from build123d import *

# Parameters (mm, degrees)
BOSS_EXTRUDE1_DEPTH = 50.8
CUT_EXTRUDE1_REACH  = 61.906
SKETCH2_R           = 3.175
CUT_EXTRUDE2_REACH  = 61.906
SKETCH3_R           = 3.175
SKETCH4_W           = 25.4
SKETCH4_H           = 25.4
SKETCH4_R           = 3.175
BOSS_EXTRUDE2_DEPTH = 6.35


with BuildPart() as part:
    # Sketch1 → Boss-Extrude1 (new body)
    with BuildSketch(Plane.XY):
        Polygon((0, 0), (25.4, 0), (25.4, 16.852186277), (25.4, 25.4), (19.05, 25.4), (19.05, 6.35), (0, 6.35), align=None)
    extrude(amount=BOSS_EXTRUDE1_DEPTH)

    # Sketch2 → Cut-Extrude1 (cut, up to next)
    with BuildSketch(Plane(origin=(0, 6.35, 0), x_dir=(1, 0, 0), z_dir=(0, 1, 0)), mode=Mode.PRIVATE) as cut_extrude1_sk1:
        with Locations(Location((9.525, -12.7, 0), (0, 0, 180))):
            Circle(SKETCH2_R)
    cut_extrude1_tool1 = extrude(cut_extrude1_sk1.sketch, amount=-CUT_EXTRUDE1_REACH, mode=Mode.PRIVATE) & part.part
    # Sketch2 → Cut-Extrude1 (cut, up to next)
    with BuildSketch(Plane(origin=(0, 6.35, 0), x_dir=(1, 0, 0), z_dir=(0, 1, 0)), mode=Mode.PRIVATE) as cut_extrude1_sk2:
        with Locations(Location((9.525, -38.1, 0), (0, 0, 180))):
            Circle(SKETCH2_R)
    cut_extrude1_tool2 = extrude(cut_extrude1_sk2.sketch, amount=-CUT_EXTRUDE1_REACH, mode=Mode.PRIVATE) & part.part
    add(cut_extrude1_tool1.solids().sort_by_distance((9.525, 6.35, 12.7))[0], mode=Mode.SUBTRACT)
    add(cut_extrude1_tool2.solids().sort_by_distance((9.525, 6.35, 38.1))[0], mode=Mode.SUBTRACT)

    # Sketch3 → Cut-Extrude2 (cut, up to next)
    with BuildSketch(Plane.ZY.offset(-19.05), mode=Mode.PRIVATE) as cut_extrude2_sk1:
        with Locations((25.4, 15.875)):
            Circle(SKETCH3_R)
    cut_extrude2_tool1 = extrude(cut_extrude2_sk1.sketch, amount=-CUT_EXTRUDE2_REACH, mode=Mode.PRIVATE) & part.part
    add(cut_extrude2_tool1.solids().sort_by_distance((19.05, 15.875, 25.4))[0], mode=Mode.SUBTRACT)

    # Sketch4 → Boss-Extrude2 (add)
    with BuildSketch(Plane.ZY.offset(-19.05)):
        with Locations((25.4, 38.1)):
            Rectangle(SKETCH4_W, SKETCH4_H)
        with Locations((25.4, 38.1)):
            Circle(SKETCH4_R, mode=Mode.SUBTRACT)
    extrude(amount=-BOSS_EXTRUDE2_DEPTH)


solid = part.part
CAD build for the part. Positions are in the model's coordinates, mm. A direction names the side the tool comes from. Give positions to 0.01 mm unless a question says otherwise; leave off trailing zeros. Write each loop counter-clockwise with the first axis right and the second up, starting at its lowest first coordinate (ties: lowest second). Pieces come first, ordered by that corner, then holes. Notation, with made-up numbers: M 36.25,28 L 46.25,28 A22 cw 46.25,56 Z; hole C 12.5,24 d3. An arc over 180 degrees is marked long. Put each result on its own line as item: value. Start each with the question number.
(1) Band-saw the part on A-A, the plane y = 38.1. Write the cut outline in (x, z) (3 decimals), and give its area (3 significant figures).
(2) Which spindle directions (+Z, -Z, +X, -X, +Y, -Y) get a long thin tool onto all of the face, cutting with end or side? Do faces 4 (the face through (10, 6.35, 25)), 5 (the face through (22, 25.4, 6)), 6 (the face through (22, 25.4, 44)), 7 (the face through (12.045, 3.219, 36.168)). Say none if no direction does.
(3) Band-saw the part on C-C, the plane x = 20.75. Write the cut outline in (y, z) (3 decimals).
(4) Flat gauge pins, fed straight in: pin 1 Ø4 at (y, z) = (29.5, 14.5) entering from -X; pin 2 Ø7 at (x, z) = (21, 4) entering from +Y; pin 3 Ø8 at (x, z) = (5, 29) entering from +Y. Where does each tip first touch, or does it go through?
(5) Band-saw the part on B-B, the plane z = 25.4. Write the cut outline in (x, y) (3 decimals).
(6) Band-saw the part on D-D, the plane z = 14.5. Write the cut outline in (x, y).
(7) Probe L1, parallel to Y at x = 21.5, z = 25.4 (3 decimals); L2, parallel to X at y = 5, z = 38; L3, parallel to Y at x = 22.5, z = 4.5. List the from-to ranges inside material, lowest first.
(8) Mould opens along X. For faces 1 (the face through (22.18, 16.83, 28.43)), 2 (the face through (25.4, 19.4, 25)), 3 (the face through (12.045, 3.219, 10.768)) say: +X half, -X half, draft (parallel to the pull), parting line (faces both ways), or undercut.
Response values:
1. outline: M 19.05,12.7 L 25.4,12.7 L 25.4,22.225 L 19.05,22.225 Z; M 19.05,28.575 L 25.4,28.575 L 25.4,38.1 L 19.05,38.1 Z
1. area: 121 mm2
2. face 4: +Z, -Z, -X, +Y
2. face 5: -Z, +X, -X, +Y
2. face 6: +Z, +X, -X, +Y
2. face 7: +Y, -Y
3. outline: M 0,0 L 25.4,0 L 25.4,12.7 L 50.8,12.7 L 50.8,38.1 L 25.4,38.1 L 25.4,50.8 L 0,50.8 Z; hole C 15.875,25.4 d6.35; hole C 38.1,25.4 d6.35
4. pin 1: stops at x = 19.05
4. pin 2: stops at y = 25.4
4. pin 3: stops at y = 6.35
5. outline: M 0,0 L 25.4,0 L 25.4,12.7 L 19.05,12.7 L 19.05,6.35 L 0,6.35 Z; M 19.05,19.05 L 25.4,19.05 L 25.4,34.925 L 19.05,34.925 Z; M 19.05,41.275 L 25.4,41.275 L 25.4,50.8 L 19.05,50.8 Z
6. outline: M 0,0 L 6.91,0 L 6.91,6.35 L 0,6.35 Z; M 12.14,0 L 25.4,0 L 25.4,50.8 L 19.05,50.8 L 19.05,6.35 L 12.14,6.35 Z
7. L1: y = 0 to 12.7, 19.05 to 34.925, 41.275 to 50.8
7. L2: x = 0 to 6.35, 12.7 to 25.4
7. L3: y = 0 to 25.4
8. face 1: draft
8. face 2: +X half
8. face 3: undercut
